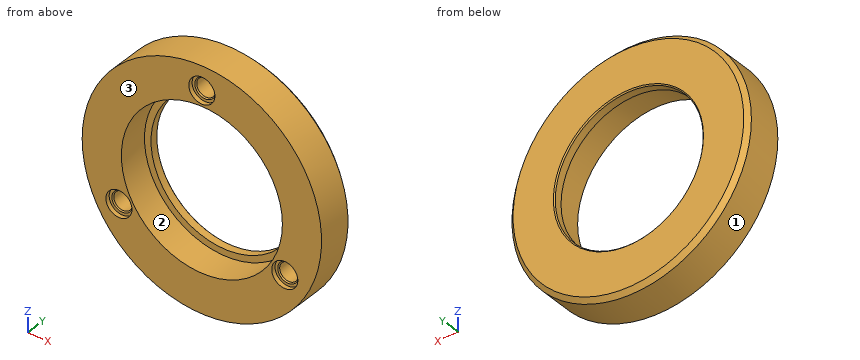
Autodesk Inventor part; units mm, degrees
ref_plane "YZ Plane" through (0, 0, 0) normal (1, 0, 0) x (0, 1, 0)
ref_plane "XZ Plane" through (0, 0, 0) normal (0, 1, 0) x (-1, 0, 0)
ref_plane "XY Plane" through (0, 0, 0) normal (0, 0, 1) x (1, 0, 0)
sketch "Sketch1" plane through (0, 0, 0) normal (0, 1, 0) x (-1, 0, 0)
  circle A0 centre (0, 0) radius 27.5
  dimension "d0" = 55
extrude "Extrusion1" add sketch "Sketch1" along normal blind 9
sketch "Sketch2" plane through (0, 9, 0) normal (0, 1, 0) x (1, 0, 0)
  circle A0 centre (0, 0) radius 17
  dimension "d3" = 34
extrude "Extrusion2" cut sketch "Sketch2" against normal through all
sketch "Sketch3" plane through (0, 0, 0) normal (0, -1, 0) x (1, 0, 0)
  circle A0 centre (0, 0) radius 18.5
  dimension "d6" = 37
extrude "Extrusion3" cut sketch "Sketch3" against normal blind 7
chamfer "Chamfer1" distance 1 angle 45 1 edges at (27.5, 9, 0)
sketch "Sketch4" plane through (0, 0, 0) normal (0, -1, 0) x (1, 0, 0)
  line L0 (0, 0) -> (0, 22)
  circle A0 centre (0, 22) radius 2.125
  circle A1 centre (-19.0526, -11) radius 2.125
  circle A2 centre (19.0526, -11) radius 2.125
  dimension "d12" = 22
  dimension "d13" = 4.25
  dimension "d16" = 360
extrude "Extrusion4" cut sketch "Sketch4" against normal blind 6.5
chamfer "Chamfer3" distance 0.25 angle 45 1 edges at (-17, 9, 0)
sketch "Sketch5" plane through (0, 0, 0) normal (0, -1, 0) x (1, 0, 0)
  circle A0 centre (0, 22) radius 2.125
  circle A1 centre (0, 22) radius 3
  circle A2 centre (19.0526, -11) radius 2.125
  circle A3 centre (19.0526, -11) radius 3
  circle A4 centre (-19.0526, -11) radius 2.125
  circle A5 centre (-19.0526, -11) radius 3
  point P0 (0, 0)
  dimension "d26" = 6
  dimension "d27" = 6
  dimension "d28" = 6
extrude "Extrusion5" cut sketch "Sketch5" against normal blind 1 contours A1 | A2 | A3 | A4 | A5
chamfer "Chamfer7" distance 0.25 angle 45 3 edges at (-2.125, 1, 22) (16.9276, 1, -11) (-21.1776, 1, -11)
properties part number "Bearing_Holder" material "ABS Plastic"
Input: part model. Units: mm. Frame: model coordinates. Face numbers are marked on the shaded views. Round coordinates to 2 decimals unless told otherwise and drop trailing zeros. Loops run counter-clockwise (first coordinate to the right, second up) from the corner with the lowest first, then second, coordinate; pieces in that order, holes last. Notation, with made-up numbers: M 45,88.25 L 64,88.25 A25 ccw 64,112.25 Z; hole C 56,3.25 d6. An arc over 180 degrees is marked long. Answer as CSV lines item,"result". Start each with the question number.
(1) First-contact query: pin 1 (2 mm diameter, centred on x = -19, z = -12, fed in from -Y); pin 2 (5 mm diameter, centred on x = -19.05, z = -11, fed in from -Y); pin 3 (8 mm diameter, centred on x = -11.5, z = 0.5, fed in from -Y); pin 4 (3 mm diameter, centred on y = 8, z = 2.5, fed in from -X). Flat tips, straight axial feed; report the tip coordinate or a pass-through.
(2) Line query: line 1 (Z direction, x = 0, y = 4) (3 decimals); line 2 (X direction, y = 1.75, z = -11.5); line 3 (X direction, y = 6.25, z = -1). Output: solid intervals per line, ascending. Write a range as [from, to].
(3) Section A-A, the plane x = 0. Output: boundary loops of the cut face in (y, z) (3 decimals), plus the area to 4 significant figures.
(4) Section C-C, the plane y = 5.5. Output: boundary loops of the cut face in (x, z) (3 decimals), plus the area to 3 significant figures.
(5) Draft query along Z for the marked faces 1, 2 and 3. Return one class per face: released by +Z, released by -Z, zero draft, split by the parting line, or undercut.
(6) Section B-B, the plane z = 0. Output: boundary loops of the cut face in (x, y).
Values found:
1,pin 1,"stops at y = 6.5"
1,pin 2,"stops at y = 1"
1,pin 3,"passes through"
1,pin 4,"stops at x = -27.48"
2,line 1,"z = [-27.5, -18.5], [18.5, 19.875], [24.125, 27.5]"
2,line 2,"x = [-24.98, -21.12], [-16.99, -14.49], [14.49, 16.99], [21.12, 24.98]"
2,line 3,"x = [-27.48, -18.47], [18.47, 27.48]"
3,outline,"M 0,-27.5 L 8,-27.5 L 9,-26.5 L 9,-17.25 L 8.75,-17 L 7,-17 L 7,-18.5 L 0,-18.5 Z; M 0,18.5 L 7,18.5 L 7,17 L 8.75,17 L 9,17.25 L 9,26.5 L 8,27.5 L 0,27.5 L 0,25 L 1,25 L 1,24.375 L 1.25,24.125 L 6.5,24.125 L 6.5,19.875 L 1.25,19.875 L 1,19.625 L 1,19 L 0,19 Z"
3,area,"137.5 mm²"
4,outline,"C 0,0 d55; hole C -19.053,-11 d4.25; hole C 0,0 d37; hole C 0,22 d4.25; hole C 19.053,-11 d4.25"
4,area,"1,260 mm²"
5,face 1,"split by the parting line"
5,face 2,"undercut"
5,face 3,"zero draft"
6,outline,"M -27.5,0 L -18.5,0 L -18.5,7 L -17,7 L -17,8.75 L -17.25,9 L -26.5,9 L -27.5,8 Z; M 17,7 L 18.5,7 L 18.5,0 L 27.5,0 L 27.5,8 L 26.5,9 L 17.25,9 L 17,8.75 Z"
